Autodesk Inventor part; units mm, degrees
ref_plane "YZ Plane" through (0, 0, 0) normal (1, 0, 0) x (0, 1, 0)
ref_plane "XZ Plane" through (0, 0, 0) normal (0, 1, 0) x (-1, 0, 0)
ref_plane "XY Plane" through (0, 0, 0) normal (0, 0, 1) x (1, 0, 0)
sketch "Sketch1" plane through (0, 0, 0) normal (0, 0, 1) x (1, 0, 0)
  line L0 (0, 0) -> (80, 0)
  line L1 (80, 0) -> (80, 53)
  line L2 (0, 53) -> (0, 0)
  line L3 (30, 53) -> (30, 39)
  arc A0 (30, 39) -> (50, 39) centre (40, 39) ccw
  line L4 (50, 39) -> (50, 53)
  line L5 (80, 53) -> (50, 53)
  line L6 (30, 53) -> (0, 53)
  circle A1 centre (15, 39.5) radius 2.1
  circle A2 centre (65, 39.5) radius 2.1
  line L7 (3, 20) -> (9, 20)
  line L8 (9, 20) -> (9, 12)
  line L9 (9, 12) -> (3, 12)
  line L10 (3, 12) -> (3, 20)
  line L11 (71, 20) -> (77, 20)
  line L12 (77, 20) -> (77, 12)
  line L13 (77, 12) -> (71, 12)
  line L14 (71, 12) -> (71, 20)
  line L15 (71, 43) -> (77, 43)
  line L16 (77, 43) -> (77, 35)
  line L17 (77, 35) -> (71, 35)
  line L18 (71, 35) -> (71, 43)
  line L19 (3, 43) -> (9, 43)
  line L20 (9, 43) -> (9, 35)
  line L21 (9, 35) -> (3, 35)
  line L22 (3, 35) -> (3, 43)
  point P0 (40, 0)
  dimension "d0" = 80
  dimension "d1" = 53
  dimension "d2" = 20
  dimension "d3" = 14
  dimension "d4" = 13.5
  dimension "d5" = 4.2
  dimension "d6" = 4.2
  dimension "d9" = 8
  dimension "d10" = 6
  dimension "d11" = 8
  dimension "d12" = 15
  dimension "d13" = 3
  dimension "d14" = 12
  dimension "d15" = 8
  dimension "d16" = 8
  dimension "d17" = 6
  dimension "d18" = 3
  dimension "d19" = 50
  dimension "d20" = 15
extrude "Extrusion1" add sketch "Sketch1" along normal blind 6
sketch "Sketch2" plane through (0, 0, 6) normal (0, 0, 1) x (1, 0, 0)
  line L0 (0, 0) -> (80, 0)
  line L1 (17.75, 16.3) -> (22.25, 16.3)
  line L2 (22.25, 0) -> (17.75, 0)
  line L3 (24.75, 12.3) -> (24.75, 5)
  line L4 (15.25, 5) -> (15.25, 12.3)
  line L5 (57.75, 16.3) -> (62.25, 16.3)
  line L6 (62.25, 0) -> (57.75, 0)
  line L7 (64.75, 12.3) -> (64.75, 5)
  line L8 (55.25, 5) -> (55.25, 12.3)
  line L9 (22.25, 16.3) -> (22.25, 12.3)
  line L10 (22.25, 5) -> (22.25, 0)
  line L11 (17.75, 0) -> (17.75, 5)
  line L12 (17.75, 12.3) -> (17.75, 16.3)
  line L13 (15.25, 12.3) -> (17.75, 12.3)
  line L14 (22.25, 12.3) -> (24.75, 12.3)
  line L15 (24.75, 5) -> (22.25, 5)
  line L16 (17.75, 5) -> (15.25, 5)
  line L17 (55.25, 12.3) -> (57.75, 12.3)
  line L18 (62.25, 12.3) -> (64.75, 12.3)
  line L19 (64.75, 5) -> (62.25, 5)
  line L20 (57.75, 5) -> (55.25, 5)
  line L21 (62.25, 16.3) -> (62.25, 12.3)
  line L22 (62.25, 5) -> (62.25, 0)
  line L23 (57.75, 0) -> (57.75, 5)
  line L24 (57.75, 12.3) -> (57.75, 16.3)
  line L25 (24.75, 8.65) -> (55.25, 8.65) construction
  point P0 (20, 16.3)
  point P1 (60, 16.3)
  point P2 (40, 8.65)
  point P3 (40, 0)
  dimension "d23" = 4.5
  dimension "d24" = 5
  dimension "d25" = 7.3
  dimension "d26" = 4
  dimension "d27" = 2.5
  dimension "d28" = 2.5
  dimension "d29" = 4.5
  dimension "d30" = 5
  dimension "d31" = 4
  dimension "d32" = 7.3
  dimension "d33" = 2.5
  dimension "d34" = 2.5
  dimension "d35" = 40
extrude "Extrusion2" cut sketch "Sketch2" against normal through all
sketch "Sketch3" plane through (0, 0, 6) normal (0, 0, 1) x (1, 0, 0)
  line L0 (22.25, 0) -> (57.75, 0)
  line L1 (57.75, 16.3) -> (62.25, 16.3)
  line L2 (62.25, 0) -> (80, 0)
  line L3 (0, 0) -> (17.75, 0)
  line L4 (17.75, 16.3) -> (22.25, 16.3)
  line L5 (4.5, 0) -> (12.5, 0)
  line L6 (12.5, 0) -> (12.5, -4)
  line L7 (10.5, -6) -> (6.5, -6)
  line L8 (4.5, -4) -> (4.5, 0)
  line L9 (27.5, 0) -> (35.5, 0)
  line L10 (35.5, 0) -> (35.5, -4)
  line L11 (33.5, -6) -> (29.5, -6)
  line L12 (27.5, -4) -> (27.5, 0)
  line L13 (44.5, 0) -> (52.5, 0)
  line L14 (52.5, 0) -> (52.5, -4)
  line L15 (50.5, -6) -> (46.5, -6)
  line L16 (44.5, -4) -> (44.5, 0)
  line L17 (67.5, 0) -> (75.5, 0)
  line L18 (75.5, 0) -> (75.5, -4)
  line L19 (73.5, -6) -> (69.5, -6)
  line L20 (67.5, -4) -> (67.5, 0)
  arc A0 (4.5, -4) -> (6.5, -6) centre (6.5, -4) ccw
  arc A1 (10.5, -6) -> (12.5, -4) centre (10.5, -4) ccw
  arc A2 (27.5, -4) -> (29.5, -6) centre (29.5, -4) ccw
  arc A3 (33.5, -6) -> (35.5, -4) centre (33.5, -4) ccw
  arc A4 (44.5, -4) -> (46.5, -6) centre (46.5, -4) ccw
  arc A5 (50.5, -6) -> (52.5, -4) centre (50.5, -4) ccw
  arc A6 (67.5, -4) -> (69.5, -6) centre (69.5, -4) ccw
  arc A7 (73.5, -6) -> (75.5, -4) centre (73.5, -4) ccw
  point P0 (20, 16.3)
  point P1 (60, 16.3)
  dimension "d44" = 2
  dimension "d45" = 15
  dimension "d46" = 15
  dimension "d47" = 6
  dimension "d48" = 7.5
  dimension "d49" = 7.5
  dimension "d50" = 8
  dimension "d51" = 8
  dimension "d52" = 8
  dimension "d53" = 8
extrude "Extrusion3" add sketch "Sketch3" against normal blind 6
chamfer "Chamfer1" distance 4 angle 45 2 edges at (0, 53, 3) (80, 53, 3)
chamfer "Chamfer2" distance 2 angle 45 2 edges at (30, 53, 3) (50, 53, 3)
properties part number "x_carriage_extruder_mount"
Geometry check sheet. Reference: the model listing, model coordinates, mm. A direction names the side the tool comes from. Give positions to 0.01 mm unless a question says otherwise; leave off trailing zeros. Order: outer loops, then holes, each group sorted by start corner. A loop starts at its lowest first (then second) coordinate and runs counter-clockwise, first axis right, second up. Notation, with made-up numbers: (56, 0.5) - (100, 0.5) arc R24 ccw to (100, 21.5) - close; hole circle Ø11 at (43, 33). An arc over 180 degrees is marked (long way). Write item = value, one per line. Start each with the question number.
1) Section check B-B (x = 56.5). Enter the section's corners in (y, z), then the cut area to 3 significant figures.
2) Scan lines: L1, parallel to X at y = -1, z = 5.15; L2, parallel to X at y = 15, z = 1.95; L3, parallel to Y at x = 65, z = 3.4. Record each from-to range of solid material in increasing order.
3) Gauge pin test, flat ends, axial feed: pin 1 Ø2 at (y, z) = (-2, 3) entering from -X; pin 2 Ø1 at (x, y) = (61.5, 0.5) entering from -Z; pin 3 Ø1 at (x, z) = (36, 1) entering from +Y; pin 4 Ø1.2 at (x, z) = (56, 2) entering from -Y. Record the tip position at first contact, or that the pin passes through.
4) Draft check along X on faces 1 (the flat face through (39, 24, 0)), 2 (the flat face through (40, 0, 3)), 3 (the flat face through (4.5, -2, 3)), 4 (the flat face through (6, 35, 3)). Enter one of: released by +X, released by -X, zero draft, split by the parting line, or undercut.
5) Access from +Z, -Z, +X, -X, +Y, -Y to the whole of each face (thin tool, end or side, straight path). Record for faces 5 (the flat face through (65, 0, 3)), 6 (the flat face through (50, 45, 3)), 7 (the flat face through (56, 12.3, 3)).
6) Section check C-C (y = 3.5). Enter the section's corners in (x, z).
7) Section check D-D (z = 2.55). Count the separate pieces of the cut face and the enclosed holes in it, then the cut area to 3 significant figures.
8) Section check A-A (y = 31). Enter the section's corners in (x, z).
Geometry check:
q1.outline = (0, 0) - (5, 0) - (5, 6) - (0, 6) - close; (12.3, 0) - (53, 0) - (53, 6) - (12.3, 6) - close
q1.area = 274 mm2
q2.L1 = 4.5 to 12.5, 27.5 to 35.5, 44.5 to 52.5, 67.5 to 75.5
q2.L2 = 0 to 3, 9 to 17.75, 22.25 to 57.75, 62.25 to 71, 77 to 80
q2.L3 = 0 to 37.4, 41.6 to 53
q3.pin_1 = 4.5
q3.pin_2 = through
q3.pin_3 = 30.07
q3.pin_4 = 0
q4.face_1 = zero draft
q4.face_2 = undercut
q4.face_3 = released by -X
q4.face_4 = undercut
q5.face_5 = +Z, -Z, -Y
q5.face_6 = +Z, -Z, +Y
q5.face_7 = +Z, -Z
q6.outline = (0, 0) - (17.75, 0) - (17.75, 6) - (0, 6) - close; (22.25, 0) - (57.75, 0) - (57.75, 6) - (22.25, 6) - close; (62.25, 0) - (80, 0) - (80, 6) - (62.25, 6) - close
q7.separate_pieces = 1
q7.enclosed_holes = 6
q7.area = 3,530 mm2
q8.outline = (0, 0) - (34, 0) - (34, 6) - (0, 6) - close; (46, 0) - (80, 0) - (80, 6) - (46, 6) - close
